Input: part model. Units: mm. Frame: model coordinates. Face numbers are marked on the shaded views. A direction names the side the tool comes from. Coordinates: 2 decimals unless noted, no trailing zeros. Loops run counter-clockwise (first coordinate to the right, second up) from the corner with the lowest first, then second, coordinate; pieces in that order, holes last.
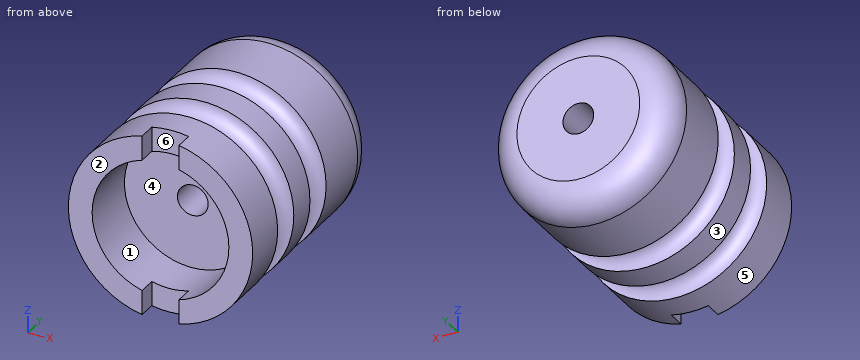
```python
from build123d import *

# Parameters (mm, degrees)
SKETCH2_R          = 5
SKETCH3_R          = 5
CUT_EXTRUDE1_DEPTH = 76
SKETCH4_R          = 22.261929886
CUT_EXTRUDE2_DEPTH = 20
SKETCH5_W          = 12
SKETCH5_H          = 6
CUT_EXTRUDE3_DEPTH = 35


with BuildPart() as part:
    # Sketch1 → Revolve1 (revolve)
    with BuildSketch(Plane.XY):
        with BuildLine():
            Line((0, -40.450423349), (0, 34.549576651))
            Line((0, 34.549576651), (20, 34.549576651))
            ThreePointArc((20, 34.549576651), (27.071067812, 31.620644463), (30, 24.549576651))
            Line((30, 24.549576651), (30, -40.450423349))
            Line((30, -40.450423349), (0, -40.450423349))
        make_face()
    revolve(axis=Axis((0, -40.450423349, 0), (0, 1, 0)))

    # Sketch2 → Cut-Revolve1 (revolve, cut)
    with BuildSketch(Plane.XY):
        with Locations((30, 0)):
            Circle(SKETCH2_R)
        with Locations((30, -20)):
            Circle(SKETCH2_R)
    revolve(axis=Axis((0, -46.378397734, 0), (0, 1, 0)), mode=Mode.SUBTRACT)

    # Sketch3 → Cut-Extrude1 (cut, through all)
    with BuildSketch(Plane(origin=(0, 34.549576651, 0), x_dir=(1, 0, 0), z_dir=(0, 1, 0))):
        Circle(SKETCH3_R)
    extrude(amount=-CUT_EXTRUDE1_DEPTH, mode=Mode.SUBTRACT)

    # Sketch4 → Cut-Extrude2 (cut)
    with BuildSketch(Plane.XZ.offset(40.450423349)):
        Circle(SKETCH4_R)
    extrude(amount=-CUT_EXTRUDE2_DEPTH, mode=Mode.SUBTRACT)

    # Sketch5 → Cut-Extrude3 (cut, symmetric)
    with BuildSketch(Plane.XY):
        with Locations((0, -37.450423349)):
            Rectangle(SKETCH5_W, SKETCH5_H)
    extrude(amount=CUT_EXTRUDE3_DEPTH, both=True, mode=Mode.SUBTRACT)


solid = part.part
```
Item 1: Section query C-C (y = -31). Output: boundary loops of the cut face in (x, z).
Result:
outline: circle Ø60 at (0, 0); hole circle Ø44.52 at (0, 0)
Item 2: Contact query for flat-ended pins moving along their axis: P1, Ø3, axis at x = -8.5, z = 5.5, coming from the -Y side; P2, Ø2, axis at x = -24, y = -14.5, coming from the +Z side; P3, Ø5, axis at y = -38, z = 24, coming from the +X side; P4, Ø8, axis at x = 0, z = 0, coming from the +Y side. Output: stop coordinate, or through.
Result:
P1: stops at y = -20.45
P2: stops at z = 19.26
P3: stops at x = 20.92
P4: passes through
Item 3: Section query D-D (y = 13). Output: boundary loops of the cut face in (x, z).
Result:
outline: circle Ø60 at (0, 0); hole circle Ø10 at (0, 0)
Item 4: Section query A-A (x = 0). Output: boundary loops of the cut face in (y, z), then the cut area to 3 significant figures.
Result:
outline: (-34.45, -30) - (-25, -30) arc R5 cw to (-15, -30) - (-5, -30) arc R5 cw to (5, -30) - (24.55, -30) arc R10 ccw to (34.55, -20) - (34.55, -5) - (-20.45, -5) - (-20.45, -22.26) - (-34.45, -22.26) - close; (-34.45, 22.26) - (-20.45, 22.26) - (-20.45, 5) - (34.55, 5) - (34.55, 20) arc R10 ccw to (24.55, 30) - (5, 30) arc R5 cw to (-5, 30) - (-15, 30) arc R5 cw to (-25, 30) - (-34.45, 30) - close
area: 2,770 mm2
Item 5: Section query B-B (z = 0). Output: boundary loops of the cut face in (x, y), then the cut area to 3 significant figures.
Result:
outline: (-30, -40.45) - (-22.26, -40.45) - (-22.26, -20.45) - (-5, -20.45) - (-5, 34.55) - (-20, 34.55) arc R10 ccw to (-30, 24.55) - (-30, 5) arc R5 cw to (-30, -5) - (-30, -15) arc R5 cw to (-30, -25) - close; (5, -20.45) - (22.26, -20.45) - (22.26, -40.45) - (30, -40.45) - (30, -25) arc R5 cw to (30, -15) - (30, -5) arc R5 cw to (30, 5) - (30, 24.55) arc R10 ccw to (20, 34.55) - (5, 34.55) - close
area: 2,860 mm2
Item 6: Reachability of the marked faces 4, 5 and 6 from +Z, -Z, +X, -X, +Y, -Y: full face, straight path, thin tool, end or side. Return the list, or none.
Result:
face 4: -Y
face 5: +Y, -Y
face 6: +Z, -Z, -Y
Item 7: Line query: L1, parallel to X at y = -34, z = 0; L2, parallel to X at y = 21, z = 0. Output: solid intervals per line, ascending.
Result:
L1: x = -30 to -22.26, 22.26 to 30
L2: x = -30 to -5, 5 to 30
Item 8: Mould query, pull axis X, two halves, no side actions, for the marked faces 1, 2 and 3. Classes: +X half, -X half, draft (parallel to the pull), parting line (faces both ways), or undercut.
Result:
face 1: undercut
face 2: draft
face 3: parting line
